from build123d import *

# Parameters (mm, degrees)
BASE_APPROXIMATE_DEPTH       = 30.6324
BEAM_CHANNEL_CROSS_SECTION_W = 38.1
BEAM_CHANNEL_CROSS_SECTION_H = 12.7
BEAM_CHANNEL_DEPTH           = 64.5
BEAM_CHANNEL_DEPTH_BACK      = 64.5
HOLE_CROSS_SECTION_R         = 19.05
HOLE_DEPTH                   = 25.4
ROUND_PART_CROSS_SECTION_R   = 44.45
ROUND_PART_DEPTH             = 81.153


with BuildPart() as part:
    # Base → Base Approximate (new body, symmetric)
    with BuildSketch(Plane(origin=(0, 0, 0), x_dir=(1, 0, 0), z_dir=(0, 1, 0))):
        Polygon((0, -63.5), (0, 63.5), (38.1, 63.5), (88.9, 44.45), (88.9, -44.45), (38.1, -63.5), align=None)
    extrude(amount=BASE_APPROXIMATE_DEPTH, both=True)

    # Beam Channel Cross Section → Beam Channel (cut, two sides)
    with BuildSketch(Plane.XY) as beam_channel_sk:
        with Locations((19.05, 0)):
            Rectangle(BEAM_CHANNEL_CROSS_SECTION_W, BEAM_CHANNEL_CROSS_SECTION_H)
    extrude(amount=BEAM_CHANNEL_DEPTH, mode=Mode.SUBTRACT)
    extrude(beam_channel_sk.sketch, amount=-BEAM_CHANNEL_DEPTH_BACK, mode=Mode.SUBTRACT)

    # Hole Cross Section → Hole (cut)
    with BuildSketch(Plane(origin=(0, 30.6324, 0), x_dir=(1, 0, 0), z_dir=(0, 1, 0))):
        with Locations((63.5, 0)):
            Circle(HOLE_CROSS_SECTION_R)
    extrude(amount=-HOLE_DEPTH, mode=Mode.SUBTRACT)

    # Round Part Cross Section → Round Part (add)
    with BuildSketch(Plane(origin=(0, 30.6324, 0), x_dir=(1, 0, 0), z_dir=(0, 1, 0))):
        with Locations((63.5, 0)):
            Circle(ROUND_PART_CROSS_SECTION_R)
    extrude(amount=ROUND_PART_DEPTH)


solid = part.part
Model file for the job. Use its own axes, mm. A direction names the side the tool comes from. Give positions to 0.01 mm unless a question says otherwise; leave off trailing zeros. Loops run counter-clockwise (first coordinate to the right, second up) from the corner with the lowest first, then second, coordinate; pieces in that order, holes last. Notation, with made-up numbers: (60.5, -4.75) -> (108.5, -4.75) arc R9 cw to (108.5, 5.25) -> close; hole circle Ø3 at (81, 7.25). An arc over 180 degrees is marked (long way). Use a Markdown table: item, result. Add a question column.
(1) Tool access for faces 4 (the flat face through (96, 30.632, -1)), 5 (the flat face through (63, 30.632, 0)), 6 (the flat face through (19, 6.35, -1)): list every direction of +Z, -Z, +X, -X, +Y, -Y with a clear straight run to the whole face (end or side of a thin tool).
(2) Mould opens along X. For faces 1 (the flat face through (63, 111.785, -1)), 2 (the cylindrical face through (105.897, 70.641, -13.352)), 3 (the flat face through (63, 5.232, 0)) say: +X half, -X half, draft (parallel to the pull), parting line (faces both ways), or undercut.
(3) Slice it at C-C on y = 26. List the corners of the cut face in (x, z), and give its area (3 significant figures).
(4) Wall check: line 1 along X through (y, z) = (19.5, 0); line 2 along Y through (x, z) = (10, -36); line 3 along Y through (x, z) = (63.5, 13.5). Give the ranges that are in metal, low to high.
(5) Drop flat-ended pins along their axis: pin 1 Ø5 at (y, z) = (36, -36.5) entering from +X; pin 2 Ø4 at (y, z) = (1.5, 28.5) entering from -X; pin 3 Ø10 at (y, z) = (39, -3) entering from -X. Give the stop position or say it passes through.
(6) Slice it at B-B on z = 0. List the corners of the cut face in (x, y), and give its area (3 significant figures).
(7) Slice it at D-D on z = 48.5. List the corners of the cut face in (x, y), and give its area (3 significant figures).
(8) Slice it at A-A on x = 13. List the corners of the cut face in (y, z), and give its area (3 significant figures).
Filled sheet:
| question | item | result |
|---|---|---|
| 1 | face 4 | +Z, -Z, +X, -Y |
| 1 | face 5 | none |
| 1 | face 6 | +Z, -Z, -X |
| 2 | face 1 | draft |
| 2 | face 2 | parting line |
| 2 | face 3 | undercut |
| 3 | outline | (0, -63.5) -> (38.1, -63.5) -> (88.9, -44.45) -> (88.9, 44.45) -> (38.1, 63.5) -> (0, 63.5) -> close; hole circle Ø38.1 at (63.5, 0) |
| 3 | area | 9,180 mm2 |
| 4 | line 1 | 0 to 44.45, 82.55 to 88.9 |
| 4 | line 2 | -30.63 to -6.35, 6.35 to 30.63 |
| 4 | line 3 | -30.63 to 5.23, 30.63 to 111.79 |
| 5 | pin 1 | x = 92.13 |
| 5 | pin 2 | x = 38.1 |
| 5 | pin 3 | x = 19.05 |
| 6 | outline | (0, -30.63) -> (88.9, -30.63) -> (88.9, 30.63) -> (107.95, 30.63) -> (107.95, 111.79) -> (19.05, 111.79) -> (19.05, 30.63) -> (0, 30.63) -> (0, 6.35) -> (38.1, 6.35) -> (38.1, -6.35) -> (0, -6.35) -> close; hole (44.45, 5.23) -> (82.55, 5.23) -> (82.55, 30.63) -> (44.45, 30.63) -> close |
| 6 | area | 11,200 mm2 |
| 7 | outline | (0, -30.63) -> (78.1, -30.63) -> (78.1, 30.63) -> (0, 30.63) -> (0, 6.35) -> (38.1, 6.35) -> (38.1, -6.35) -> (0, -6.35) -> close |
| 7 | area | 4,300 mm2 |
| 8 | outline | (-30.63, -63.5) -> (-6.35, -63.5) -> (-6.35, 63.5) -> (-30.63, 63.5) -> close; (6.35, -63.5) -> (30.63, -63.5) -> (30.63, 63.5) -> (6.35, 63.5) -> close |
| 8 | area | 6,170 mm2 |
